Verification items for this drawing (mm, ordinates from the low corner). A direction names the side the tool comes from. Round coordinates to 2 decimals unless told otherwise and drop trailing zeros. Write each loop counter-clockwise with the first axis right and the second up, starting at its lowest first coordinate (ties: lowest second). Pieces come first, ordered by that corner, then holes. Notation, with made-up numbers: (-8.5, -11.5) -> (4.5, -11.5) arc R21 cw to (4.5, 24.5) -> close; hole circle Ø4 at (59, -33.5). An arc over 180 degrees is marked (long way). Put each result on its own line as item: value. Start each with the question number.
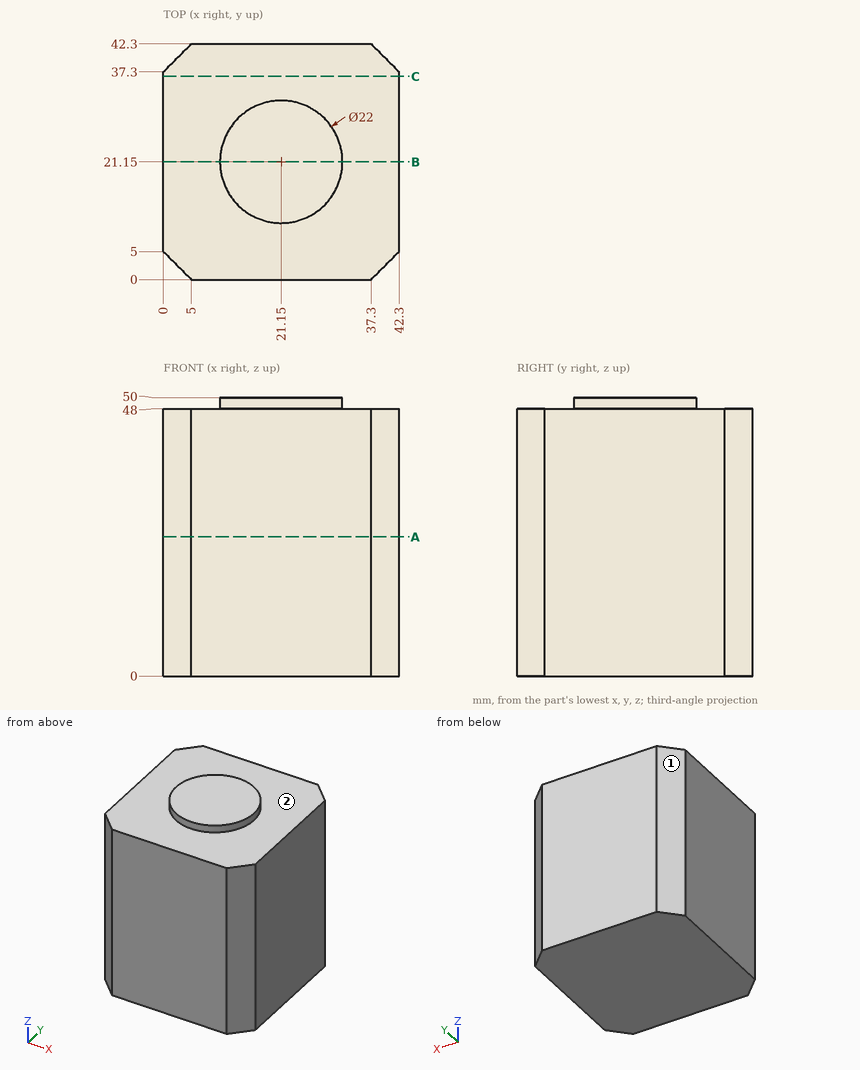
1. Material ranges on L1, parallel to Z at x = 36.5, y = 4; L2, parallel to X at y = 2.5, z = 46; L3, parallel to X at y = 39.5, z = 23.5, recorded low to high. Write a range as [from, to].
2. Section check B-B, the plane y = 21.15. Enter the section's corners in (x, z).
3. Gauge pin test, flat end, axial feed: P1, Ø8, axis at x = 27, z = 25.5, coming from the -Y side. Record the tip position at first contact, or that the pin passes through.
4. Section check A-A, the plane z = 25. Enter the section's corners in (x, y), then the cut area to 3 significant figures.
5. Section check C-C, the plane y = 36.5. Enter the section's corners in (x, z).
6. Access from +Z, -Z, +X, -X, +Y, -Y to the whole of each face (thin tool, end or side, straight path). Record for the marked faces 1 and 2.
Reply:
1. L1: z = [0, 48]
1. L2: x = [2.5, 39.8]
1. L3: x = [2.2, 40.1]
2. outline: (0, 0) -> (42.3, 0) -> (42.3, 48) -> (32.15, 48) -> (32.15, 50) -> (10.15, 50) -> (10.15, 48) -> (0, 48) -> close
3. P1: stops at y = 0
4. outline: (0, 5) -> (5, 0) -> (37.3, 0) -> (42.3, 5) -> (42.3, 37.3) -> (37.3, 42.3) -> (5, 42.3) -> (0, 37.3) -> close
4. area: 1,740 mm2
5. outline: (0, 0) -> (42.3, 0) -> (42.3, 48) -> (0, 48) -> close
6. face 1: +Z, -Z, -X, +Y
6. face 2: +Z
